Source: CAD feature listing. Evaluate the final solid. Frame: model axes, mm. Face numbers are marked on the shaded views. A direction names the side the tool comes from. Round coordinates to 2 decimals unless told otherwise and drop trailing zeros. Write each loop counter-clockwise with the first axis right and the second up, starting at its lowest first coordinate (ties: lowest second). Pieces come first, ordered by that corner, then holes. Notation, with made-up numbers: M 17.5,33 L 74.5,33 A21 ccw 74.5,54 Z; hole C -19.75,63.5 d1. An arc over 180 degrees is marked long. Answer in a Markdown table with one row per item. Add a question column.
Item 1: Cut plane A-A on z = 30.5. Return loops of the section in (x, y).
Item 2: Contact query for a flat-ended pin moving along its axis: pin 1 (12 mm diameter, centred on x = 15, z = 44, fed in from +Y). Output: stop coordinate, or through.
Item 3: Cut plane C-C on z = 43.5. Return loops of the section in (x, y).
Item 4: Set-up query: the marked faces 1 and 2. Return all of +Z, -Z, +X, -X, +Y, -Y with unobstructed straight access to the full face (end or side cutting, diameter ignored); none if empty.
Item 5: Cut plane B-B on y = 10. Return loops of the section in (x, z).
Item 6: Material intervals for probe 1 along X at (y, z) = (15.25, 50); probe 2 along X at (y, z) = (2, 49.5), sorted ascending.
Item 7: Cut plane D-D on x = 7.25. Return loops of the section in (y, z).
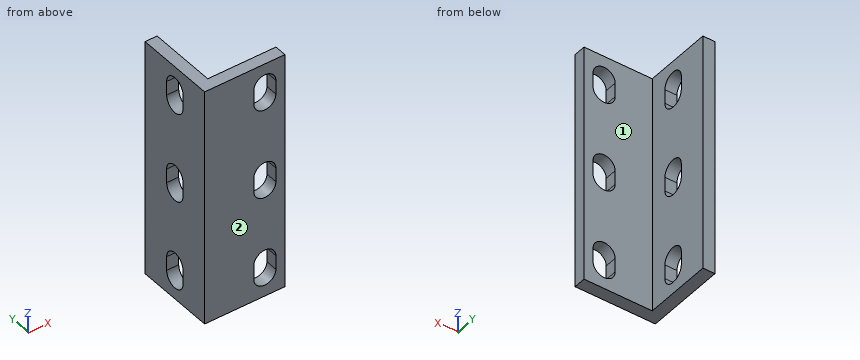
from build123d import *

# Parameters (mm, degrees)
EXTRUDE_THIN1_DEPTH = 59.6
CUT_EXTRUDE1_DEPTH  = 4
CUT_EXTRUDE2_DEPTH  = 4


with BuildPart() as part:
    # Sketch1 → Extrude-Thin1 (new body)
    with BuildSketch(Plane.XY):
        Polygon((0, 20), (0, 0), (20, 0), (20, 3), (3, 3), (3, 20), align=None)
    extrude(amount=EXTRUDE_THIN1_DEPTH)

    # Sketch2 → Cut-Extrude1 (cut, through all)
    with BuildSketch(Plane(origin=(3, 0, 0), x_dir=(0, 0, -1), z_dir=(1, 0, 0))):
        with BuildLine():
            Line((-50.55, 7.25), (-54.05, 7.25))
            ThreePointArc((-54.05, 7.25), (-56.8, 10), (-54.05, 12.75))
            Line((-54.05, 12.75), (-50.55, 12.75))
            ThreePointArc((-50.55, 12.75), (-47.8, 10), (-50.55, 7.25))
        make_face()
        with BuildLine():
            Line((-9.05, 7.25), (-5.55, 7.25))
            ThreePointArc((-5.55, 7.25), (-2.8, 10), (-5.55, 12.75))
            Line((-5.55, 12.75), (-9.05, 12.75))
            ThreePointArc((-9.05, 12.75), (-11.8, 10), (-9.05, 7.25))
        make_face()
        with BuildLine():
            Line((-28.05, 7.25), (-31.55, 7.25))
            ThreePointArc((-31.55, 7.25), (-34.3, 10), (-31.55, 12.75))
            Line((-31.55, 12.75), (-28.05, 12.75))
            ThreePointArc((-28.05, 12.75), (-25.3, 10), (-28.05, 7.25))
        make_face()
    extrude(amount=-CUT_EXTRUDE1_DEPTH, mode=Mode.SUBTRACT)

    # Sketch3 → Cut-Extrude2 (cut, through all)
    with BuildSketch(Plane(origin=(0, 3, 0), x_dir=(1, 0, 0), z_dir=(0, 1, 0))):
        with BuildLine():
            Line((12.25, -54.05), (12.25, -50.55))
            ThreePointArc((12.25, -50.55), (15, -47.8), (17.75, -50.55))
            Line((17.75, -50.55), (17.75, -54.05))
            ThreePointArc((17.75, -54.05), (15, -56.8), (12.25, -54.05))
        make_face()
        with BuildLine():
            Line((12.25, -5.55), (12.25, -9.05))
            ThreePointArc((12.25, -9.05), (15, -11.8), (17.75, -9.05))
            Line((17.75, -9.05), (17.75, -5.55))
            ThreePointArc((17.75, -5.55), (15, -2.8), (12.25, -5.55))
        make_face()
        with BuildLine():
            Line((17.75, -28.05), (17.75, -31.55))
            ThreePointArc((17.75, -31.55), (15, -34.3), (12.25, -31.55))
            Line((12.25, -31.55), (12.25, -28.05))
            ThreePointArc((12.25, -28.05), (15, -25.3), (17.75, -28.05))
        make_face()
    extrude(amount=-CUT_EXTRUDE2_DEPTH, mode=Mode.SUBTRACT)


solid = part.part
Results below:
| question | item | result |
|---|---|---|
| 1 | outline | M 0,0 L 12.25,0 L 12.25,3 L 3,3 L 3,7.25 L 0,7.25 Z; M 0,12.75 L 3,12.75 L 3,20 L 0,20 Z; M 17.75,0 L 20,0 L 20,3 L 17.75,3 Z |
| 2 | pin 1 | y = 3 |
| 3 | outline | M 0,0 L 20,0 L 20,3 L 3,3 L 3,20 L 0,20 Z |
| 4 | face 1 | +Z, -Z, +X, +Y |
| 4 | face 2 | +Z, -Z, +X, -X, -Y |
| 5 | outline | M 0,0 L 3,0 L 3,2.8 L 0,2.8 Z; M 0,11.8 L 3,11.8 L 3,25.3 L 0,25.3 Z; M 0,34.3 L 3,34.3 L 3,47.8 L 0,47.8 Z; M 0,56.8 L 3,56.8 L 3,59.6 L 0,59.6 Z |
| 6 | probe 1 | 0 to 3 |
| 6 | probe 2 | 0 to 12.46, 17.54 to 20 |
| 7 | outline | M 0,0 L 3,0 L 3,59.6 L 0,59.6 Z |
